The listing builds one solid part. Answer for the finished solid, in the listing's coordinates (mm). A direction names the side the tool comes from. Give positions to 0.01 mm unless a question says otherwise; leave off trailing zeros. Loops run counter-clockwise (first coordinate to the right, second up) from the corner with the lowest first, then second, coordinate; pieces in that order, holes last.
Item 1: Section C-C, the plane y = 1 is taken. Give the vertices of the cut face in (x, z).
Item 2: Section A-A, the plane y = -3 is taken. Give the vertices of the cut face in (x, z).
Item 3: Consider line 1 along Y through (x, z) = (0, 23.35); line 2 along Y through (x, z) = (2.25, 2); line 3 along Z through (x, y) = (-2.5, 2.5). Determine where each line is inside the solid, lowest interval first.
Item 4: Each of these flat-tipped pins is pushed along its axis until it touches: pin 1 Ø3.5 at (x, z) = (1, 5.5) entering from -Y; pin 2 Ø2 at (x, z) = (-1, 8) entering from +Y; pin 3 Ø2 at (x, y) = (2, -4) entering from -Z; pin 4 Ø2.5 at (x, z) = (-1, -16.25) entering from -Y. Where does it stop, or does it pass through?
Item 5: Section D-D, the plane x = 2 is taken. Give the vertices of the cut face in (y, z), and give its area (3 significant figures).
Item 6: A tool of negligible diameter and unlimited length cuts with its end or side. For faces 5 (the face through (2.6, 7.64, 22.98)), 6 (the face through (-2, 5, 21.5)), 7 (the face through (0, 0, 0)), from which of +Z, -Z, +X, -X, +Y, -Y can it reach the whole face along a straight path? Write none if from no direction.
Item 7: Section B-B, the plane z = -6.75 is taken. Give the vertices of the cut face in (x, y).
Item 8: The mould has two halves that part along Y. Classify faces 1 (the face through (0, 1, -21.5)), 2 (the face through (0.336, -1.487, 22.979)), 3 (the face through (2.6, -5.64, 22.98)), 4 (the face through (-2.64, 7.6, 22.98)): pulls with the +Y half, pulls with the -Y half, needs draft (parallel to the pull), parting line crosses it, or undercut.
from build123d import *

# Parameters (mm, degrees)
SKETCH_1_W           = 7
SKETCH_1_H           = 43
SKETCH_1_R           = 1.3
EXTRUDE_1_DEPTH      = 2
EXTRUDE_2_DEPTH      = 8.5
EXTRUDE_2_DEPTH_BACK = 6.5
SKETCH_2_W           = 7
SKETCH_2_H           = 3
SKETCH_3_R           = 1.55
CUT_EXTRUDE_1_DEPTH  = 27.167728216
FILLET_1_R           = 3
FILLET_2_R           = 3


with BuildPart() as part:
    # 草图1 → 凸台-拉伸1 (new body)
    with BuildSketch(Plane(origin=(0, 0, 0), x_dir=(1, 0, 0), z_dir=(0, 1, 0))):
        Rectangle(SKETCH_1_W, SKETCH_1_H)
        with Locations(Location((-1, 16.25, 0), (0, 0, 270))):
            Circle(SKETCH_1_R, mode=Mode.SUBTRACT)
        with Locations(Location((-1, 6.75, 0), (0, 0, 90))):
            Circle(SKETCH_1_R, mode=Mode.SUBTRACT)
    extrude(amount=EXTRUDE_1_DEPTH)

    # 草图2 → 凸台-拉伸2 (add, two sides: drawn at the far end of the back side and taken through both)
    with BuildSketch(Plane(origin=(0, 0, 0), x_dir=(1, 0, 0), z_dir=(0, 1, 0)).offset(-EXTRUDE_2_DEPTH_BACK)):
        with Locations((0, -23)):
            Rectangle(SKETCH_2_W, SKETCH_2_H)
    extrude(amount=EXTRUDE_2_DEPTH + EXTRUDE_2_DEPTH_BACK)

    # 草图3 → 切除-拉伸1 (cut, through all)
    with BuildSketch(Plane.XY):
        with Locations(Location((0, 5, 0), (0, 0, 180))):
            Circle(SKETCH_3_R)
        with Locations(Location((0, -3, 0), (0, 0, 180))):
            Circle(SKETCH_3_R)
    extrude(amount=CUT_EXTRUDE_1_DEPTH, mode=Mode.SUBTRACT)

    # 圆角1
    fillet_1_edges = [part.edges().sort_by_distance(p)[0] for p in [
        (-3.5, 1, -21.5),
        (3.5, 1, -21.5),
    ]]
    fillet(fillet_1_edges, radius=FILLET_1_R)

    # 圆角2
    fillet_2_edges = [part.edges().sort_by_distance(p)[0] for p in [
        (3.5, -6.5, 23),
        (-3.5, -6.5, 23),
        (3.5, 8.5, 23),
        (-3.5, 8.5, 23),
    ]]
    fillet(fillet_2_edges, radius=FILLET_2_R)


solid = part.part
Worked answers:
1. outline: (-3.5, -18.5) arc R3 ccw to (-0.5, -21.5) - (0.5, -21.5) arc R3 ccw to (3.5, -18.5) - (3.5, 24.5) - (-3.5, 24.5) - close; hole circle Ø2.6 at (-1, -16.25); hole circle Ø2.6 at (-1, -6.75)
2. outline: (-3.5, 21.5) - (-1.55, 21.5) - (-1.55, 24.5) - (-3.5, 24.5) - close; (1.55, 21.5) - (3.5, 21.5) - (3.5, 24.5) - (1.55, 24.5) - close
3. line 1: y = -6.5 to -4.55, -1.45 to 3.45, 6.55 to 8.5
3. line 2: y = 0 to 2
3. line 3: z = 21.5 to 24.5
4. pin 1: stops at y = 0
4. pin 2: stops at y = 2
4. pin 3: stops at z = 21.5
4. pin 4: passes through
5. outline: (-6.1, 21.5) - (0, 21.5) - (0, -21.1) - (2, -21.1) - (2, 21.5) - (8.1, 21.5) - (8.1, 24.5) - (-6.1, 24.5) - close
5. area: 128 mm2
6. face 5: +Z, -Z, +X, +Y
6. face 6: -Z, +X, -X, +Y
6. face 7: -Z, +X, -X, -Y
7. outline: (-3.5, 0) - (-2.3, 0) - (-2.3, 2) - (-3.5, 2) - close; (0.3, 0) - (3.5, 0) - (3.5, 2) - (0.3, 2) - close
8. face 1: needs draft
8. face 2: undercut
8. face 3: pulls with the -Y half
8. face 4: pulls with the +Y half
